The model under review builds one solid part; all positions refer to its coordinate system, in mm. A direction names the side the tool comes from. Coordinates: 2 decimals unless noted, no trailing zeros. Order: outer loops, then holes, each group sorted by start corner. A loop starts at its lowest first (then second) coordinate and runs counter-clockwise, first axis right, second up. Notation, with made-up numbers: M 42.25,45 L 97.25,45 A27 cw 97.25,84 Z; hole C -4,-23.75 d4. An arc over 180 degrees is marked long. Answer as CSV lines item,"result". Start each with the question number.
Q1. The part is to be moulded in two halves that separate along Y. For faces 4 (the face through (-39.8, -70.7, 37)), 5 (the face through (-25, 66, 28)), 6 (the face through (49.952, 56.985, 34.93)), say which applies: +Y half, -Y half, draft (parallel to the pull), parting line (faces both ways), or undercut.
Q2. Consider section A-A on z = 16.5. Write out the cut boundary in (x, y).
Q3. For P1, Ø3, axis at x = 14, z = -14.5, coming from the +Y side; P2, Ø10, axis at x = -6, z = 40, coming from the +Y side; P3, Ø11, axis at x = -9.5, z = 34, coming from the +Y side; P4, Ø3, axis at x = -52.5, y = 33.35, coming from the +Z side, all flat-tipped, find the tip position at first contact; note any pin that passes through.
Q4. Wall thickness on L1, parallel to Y at x = 0, z = -12; L2, parallel to Z at x = 36.5, y = 37; L3, parallel to Y at x = 52, z = 39: over which ranges is each line inside the solid? List them lowest first. Write a range as [from, to].
Q5. Consider section D-D on z = -10. Write out the cut boundary in (x, y).
Q6. Consider section C-C on x = 0. Write out the cut boundary in (y, z), and give its area (3 significant figures).
Q7. Machinability: for faces 1 (the face through (-3, -71.5, 23)), 2 (the face through (23.846, 7.509, -13.095)), 3 (the face through (0, 66, 25)), which of the approach directions +Z, -Z, +X, -X, +Y, -Y give a long, thin tool a straight path to every point of the face, cutting with its end or side? Answer none if there is none.
Q8. Consider section B-B on x = -52.5. Write out the cut boundary in (y, z).
from build123d import *

# Parameters (mm, degrees)
ESTRUSIONE_ESTRUSIONE1_DEPTH       = 30
ESTRUSIONE_ESTRUSIONE1_DEPTH_BACK  = 55
SCHIZZO1_R                         = 25
SCHIZZO1_R_2                       = 20
ESTRUSIONE_ESTRUSIONE2_DEPTH       = 10
ESTRUSIONE_ESTRUSIONE3_DEPTH       = 10
ESTRUSIONE_ESTRUSIONE5_DEPTH       = 42.5
TAGLIO_ESTRUSIONE1_DEPTH           = 26.5
SCHIZZO3D5_R                       = 2.5
TAGLIO_ESTRUSIONE2_DEPTH           = 35.5
SCHIZZO3D6_R                       = 4
TAGLIO_ESTRUSIONE3_DEPTH           = 3
ESTRUSIONE_ESTRUSIONE10_DEPTH      = 5
TAGLIO_ESTRUSIONE4_START           = -14
TAGLIO_ESTRUSIONE4_DEPTH           = 14
TAGLIO_ESTRUSIONE7_DEPTH           = 3
ESTRUSIONE_ESTRUSIONE11_START      = 30
ESTRUSIONE_ESTRUSIONE11_OUTLINE_R  = 4
ESTRUSIONE_ESTRUSIONE11_DEPTH      = 10
ESTRUSIONE_ESTRUSIONE12_DEPTH      = 10
ESTRUSIONE_ESTRUSIONE13_DEPTH      = 10
ESTRUSIONE_ESTRUSIONE14_DEPTH      = 10
TAGLIO_ESTRUSIONE11_DEPTH          = 80
SCHIZZO3D17_R                      = 4
TAGLIO_ESTRUSIONE12_DEPTH          = 3
TAGLIO_ESTRUSIONE13_START          = 30
TAGLIO_ESTRUSIONE13_OUTLINE_R      = 2.5
TAGLIO_ESTRUSIONE13_DEPTH          = 7
ESTRUSIONE_ESTRUSIONE15_DEPTH      = 5
ESTRUSIONE_ESTRUSIONE17_DEPTH      = 37.5
ESTRUSIONE_ESTRUSIONE17_DEPTH_BACK = 37.5


# Read off the part's stored shape, not the designer's step: Estrusione-Estrusione11, Taglio-Estrusione13
with BuildPart() as part:
    # Schizzo1 → Estrusione-Estrusione1 (new, two sides: drawn at the far end of the back side and taken through both)
    with BuildSketch(Plane.XY.offset(-ESTRUSIONE_ESTRUSIONE1_DEPTH_BACK)):
        Circle(SCHIZZO1_R)
        Circle(SCHIZZO1_R_2, mode=Mode.SUBTRACT)
    extrude(amount=ESTRUSIONE_ESTRUSIONE1_DEPTH + ESTRUSIONE_ESTRUSIONE1_DEPTH_BACK)

    # Schizzo3D1 → Estrusione-Estrusione2 (add)
    with BuildSketch(Plane(origin=(-37.75, 73.5, 30), x_dir=(0.4568693936855125, -0.889533786381064, 0), z_dir=(0, 0, -1))):
        Polygon((0, 0), (34.493639223, -67.159800872), (75.600538561, -73.870637396), (146.763241471, -37.321085901), (165.255105821, 0), (130.761466598, 67.159800872), (89.654567261, 73.870637396), (18.49186435, 37.321085901), align=None)
    extrude(amount=-ESTRUSIONE_ESTRUSIONE2_DEPTH)

    # Schizzo3D2 → Estrusione-Estrusione3 (add)
    with BuildSketch(Plane(origin=(62.5, 0, 30), x_dir=(-0.9968152785361251, -0.07974522228289001, 0), z_dir=(0, 0, 1))):
        Polygon((0, 0), (0.797452223, 9.968152785), (5.781528616, 9.569426674), (4.984076393, -0.398726111), align=None)
        Polygon((125.39936204, 0), (120.415285647, 0.398726111), (119.617833424, -9.569426674), (124.601909817, -9.968152785), align=None)
    extrude(amount=-ESTRUSIONE_ESTRUSIONE3_DEPTH)

    # Schizzo3D3 → Estrusione-Estrusione5 (add)
    with BuildSketch(Plane(origin=(35.227450684, -68.5, 30), x_dir=(-0.9974912873801348, -0.0707893466612134, 0), z_dir=(0, 0, 1))):
        Polygon((0, 0), (70.278150268, -4.987456437), (70.632097001, 0), (0.353946733, 4.987456437), align=None)
    extrude(amount=-ESTRUSIONE_ESTRUSIONE5_DEPTH)

    # Schizzo3D4 → Taglio-Estrusione1 (cut)
    with BuildSketch(Plane(origin=(32.75, -68.5, -12.5), x_dir=(-1, 0, 0), z_dir=(0, 1, 0))):
        with BuildLine():
            Line((0, 0), (65.5, 0))
            ThreePointArc((65.5, 0), (32.75, 32.75), (0, 0))
        make_face()
    extrude(amount=-TAGLIO_ESTRUSIONE1_DEPTH, mode=Mode.SUBTRACT)

    # Schizzo3D5 → Taglio-Estrusione2 (cut)
    with BuildSketch(Plane(origin=(-52.5, 33.353317087, 40), x_dir=(0.8440673996564301, -0.5362370975951146, 0), z_dir=(0, 0, -1))):
        with Locations(Location((0, 0, 0), (0, 0, 147.572152721))):
            Circle(SCHIZZO3D5_R)
        with Locations(Location((88.627076964, -56.304895247, 0), (0, 0, 147.572152721))):
            Circle(SCHIZZO3D5_R)
        with Locations(Location((124.397648864, 0, 0), (0, 0, 147.572152721))):
            Circle(SCHIZZO3D5_R)
        with Locations(Location((35.7705719, 56.304895247, 0), (0, 0, 147.572152721))):
            Circle(SCHIZZO3D5_R)
    extrude(amount=TAGLIO_ESTRUSIONE2_DEPTH, mode=Mode.SUBTRACT)

    # Schizzo3D6 → Taglio-Estrusione3 (cut)
    with BuildSketch(Plane(origin=(0, 73.5, 40), x_dir=(0, -1, 0), z_dir=(0, 0, -1))):
        with Locations(Location((40.146682913, 52.5, 0), (0, 0, 270))):
            Circle(SCHIZZO3D6_R)
        with Locations(Location((40.146682913, -52.5, 0), (0, 0, 270))):
            Circle(SCHIZZO3D6_R)
        with Locations(Location((106.853317087, -52.5, 0), (0, 0, 270))):
            Circle(SCHIZZO3D6_R)
        with Locations(Location((106.853317087, 52.5, 0), (0, 0, 270))):
            Circle(SCHIZZO3D6_R)
    extrude(amount=TAGLIO_ESTRUSIONE3_DEPTH, mode=Mode.SUBTRACT)

    # Schizzo3D7 → Estrusione-Estrusione10 (add)
    with BuildSketch(Plane(origin=(35.227450684, -73.5, -12.5), x_dir=(-0.8117651174974726, 0, 0.5839840700004706), z_dir=(0, 1, 0))):
        with BuildLine():
            Line((0, 0), (2.011108045, -1.446791734))
            ThreePointArc((2.011108045, -1.446791734), (47.721893936, 6.013037572), (55.181723242, -39.697748319))
            Line((55.181723242, -39.697748319), (57.192831287, -41.144540052))
            Line((57.192831287, -41.144540052), (82.012154262, -6.644522559))
            Line((82.012154262, -6.644522559), (84.059871804, -8.117651175))
            Line((84.059871804, -8.117651175), (89.899712504, 0))
            Line((89.899712504, 0), (28.611446133, 44.090797285))
            Line((28.611446133, 44.090797285), (22.771605433, 35.97314611))
            Line((22.771605433, 35.97314611), (24.819322975, 34.500017494))
            Line((24.819322975, 34.500017494), (0, 0))
        make_face()
    extrude(amount=-ESTRUSIONE_ESTRUSIONE10_DEPTH)

    # Schizzo3D8 → Taglio-Estrusione4 (cut)
    with BuildSketch(Plane(origin=(0, -78.5, 20.25), x_dir=(-0.707106781186551, 0, -0.7071067811865441), z_dir=(0, -1, 0)).offset(TAGLIO_ESTRUSIONE4_START)):
        with BuildLine():
            ThreePointArc((0, 46.315494168), (-0.707106781, -0.707106781), (46.315494168, 0))
            ThreePointArc((46.315494168, 0), (0, 0), (0, 46.315494168))
        make_face()
    extrude(amount=TAGLIO_ESTRUSIONE4_DEPTH, mode=Mode.SUBTRACT)

    # Schizzo3D9 → Taglio-Estrusione7 (cut)
    with BuildSketch(Plane(origin=(35.227450684, -68.5, -12.5), x_dir=(-0.8562730712113632, 0, 0.5165234046180869), z_dir=(0, -1, 0))):
        with BuildLine():
            Line((0, 0), (2.121374306, 1.279661262))
            ThreePointArc((2.121374306, 1.279661262), (13.749394894, 45.407843828), (58.20726047, 35.111944264))
            Line((58.20726047, 35.111944264), (60.328634776, 36.391605526))
            Line((60.328634776, 36.391605526), (82.280879472, 0))
            Line((82.280879472, 0), (21.952244696, -36.391605526))
            Line((21.952244696, -36.391605526), (0, 0))
        make_face()
    extrude(amount=TAGLIO_ESTRUSIONE7_DEPTH, mode=Mode.SUBTRACT)

    # Estrusione-Estrusione11 outline → Estrusione-Estrusione11 (add)
    with BuildSketch(Plane.XY.offset(ESTRUSIONE_ESTRUSIONE11_START)):
        with Locations((52.5, -33.353317087)):
            Circle(ESTRUSIONE_ESTRUSIONE11_OUTLINE_R)
        with Locations((-52.5, -33.353317087)):
            Circle(ESTRUSIONE_ESTRUSIONE11_OUTLINE_R)
    extrude(amount=ESTRUSIONE_ESTRUSIONE11_DEPTH)

    # Schizzo3D11 → Estrusione-Estrusione12 (add)
    with BuildSketch(Plane(origin=(-62.5, -40, 40), x_dir=(0.9979582700578467, -0.06386932928370219, 0), z_dir=(0, 0, -1))):
        Polygon((0, 0), (0.510954634, 7.98366616), (27.158436361, 36.840627497), (26.839089715, 31.850836147), align=None)
        Polygon((102.504285751, 32.018493137), (102.184939104, 27.028701786), (124.744783757, -7.98366616), (125.255738392, 0), align=None)
    extrude(amount=ESTRUSIONE_ESTRUSIONE12_DEPTH)

    # Schizzo3D12 → Estrusione-Estrusione13 (add)
    with BuildSketch(Plane(origin=(-37.75, -78.5, 40), x_dir=(0.9932296706390209, 0.11616721294023631, 0), z_dir=(0, 0, 1))):
        Polygon((0, 0), (-9.932296706, 1.161672129), (-8.770624577, 11.093968836), (1.161672129, 9.932296706), align=None)
        Polygon((74.988840133, -8.770624577), (84.92113684, -9.932296706), (86.082808969, 0), (76.150512263, 1.161672129), align=None)
    extrude(amount=-ESTRUSIONE_ESTRUSIONE13_DEPTH)

    # Schizzo3D15 → Estrusione-Estrusione14 (add)
    with BuildSketch(Plane(origin=(-49.75, -63.712121212, 40), x_dir=(0.9860632358712049, -0.16637095558783233, 0), z_dir=(0, 0, 1))):
        Polygon((0, 0), (4.627662115, -4.074759177), (2.768690441, -4.388409339), (4.432399997, -14.249041698), (98.601439022, 1.639384561), (96.937729467, 11.500016919), (95.078757792, 11.186366757), (98.113291969, 16.553910081), (100.573565494, 1.972126472), (100.906307405, 0), (2.793015436, -16.553910081), (2.460273525, -14.581783609), align=None)
    extrude(amount=-ESTRUSIONE_ESTRUSIONE14_DEPTH)

    # Schizzo3D16 → Taglio-Estrusione11 (cut)
    with BuildSketch(Plane(origin=(-49.75, -80.5, 40), x_dir=(0.9860632358712049, 0.16637095558783233, 0), z_dir=(0, 0, 1))):
        Polygon((0, 0), (1.972126472, -0.332741911), (4.35509632, 13.790870902), (2.793015436, 16.553910081), align=None)
        Polygon((98.113291969, -16.553910081), (96.141165497, -16.22116817), (98.524135346, -2.097555357), (100.906307405, 0), align=None)
    extrude(amount=-TAGLIO_ESTRUSIONE11_DEPTH, mode=Mode.SUBTRACT)

    # Schizzo3D17 → Taglio-Estrusione12 (cut)
    with BuildSketch(Plane(origin=(0, -80.5, 40), x_dir=(-0.9847878761773714, 0.17376086709631217, 0), z_dir=(0, 0, -1))):
        with Locations(Location((41.215356952, 0, 0), (0, 0, 169.993443701))):
            Circle(SCHIZZO3D17_R)
        with Locations(Location((-38.726539684, 14.10534554, 0), (0, 0, 169.993443701))):
            Circle(SCHIZZO3D17_R)
    extrude(amount=TAGLIO_ESTRUSIONE12_DEPTH, mode=Mode.SUBTRACT)

    # Taglio-Estrusione13 outline → Taglio-Estrusione13 (cut)
    with BuildSketch(Plane.XY.offset(TAGLIO_ESTRUSIONE13_START)):
        with Locations((-40.588383838, -73.338383838)):
            Circle(TAGLIO_ESTRUSIONE13_OUTLINE_R)
        with Locations((40.588383838, -73.338383838)):
            Circle(TAGLIO_ESTRUSIONE13_OUTLINE_R)
    extrude(amount=TAGLIO_ESTRUSIONE13_DEPTH, mode=Mode.SUBTRACT)

    # Schizzo3D19 → Estrusione-Estrusione15 (add)
    with BuildSketch(Plane(origin=(0, 68.5, 30), x_dir=(0.9805806756909201, -0.19611613513818418, 0), z_dir=(0, 0, -1))):
        Polygon((0, 0), (-24.514516892, 4.902903378), (-23.533936217, 9.805806757), (25.495097568, 0), (24.514516892, -4.902903378), align=None)
    extrude(amount=ESTRUSIONE_ESTRUSIONE15_DEPTH)

    # Schizzo3D21 → Estrusione-Estrusione17 (add, two sides: drawn at the far end of the back side and taken through both)
    with BuildSketch(Plane(origin=(0, 73.5, 40), x_dir=(0, 0.4472135954999578, 0.8944271909999159), z_dir=(1, 0, 0)).offset(-ESTRUSIONE_ESTRUSIONE17_DEPTH_BACK)):
        Polygon((0, 0), (38.013155617, 0), (35.329874044, 5.366563146), (-2.683281573, 5.366563146), align=None)
    extrude(amount=ESTRUSIONE_ESTRUSIONE17_DEPTH + ESTRUSIONE_ESTRUSIONE17_DEPTH_BACK)


solid = part.part
Evaluation:
1,face 4,"undercut"
1,face 5,"draft"
1,face 6,"+Y half"
2,outline,"M -35.23,-78.5 L -16.99,-78.5 L -16.99,-71.5 L -35.23,-71.5 Z; C 0,0 d50; M 16.99,-78.5 L 35.23,-78.5 L 35.23,-71.5 L 16.99,-71.5 Z; hole C 0,0 d40"
3,P1,"stops at y = 21.65"
3,P2,"stops at y = 76"
3,P3,"stops at y = 73.5"
3,P4,"passes through"
4,L1,"y = [-25, -20], [20, 25]"
4,L2,"z = [30, 40]"
4,L3,"y = [-60.94, 29.38], [37.32, 54.21]"
5,outline,"M -35.23,-78.5 L -32.73,-78.5 L -32.73,-71.5 L -35.23,-71.5 Z; C 0,0 d50; M 32.73,-78.5 L 35.23,-78.5 L 35.23,-71.5 L 32.73,-71.5 Z; hole C 0,0 d40"
6,outline,"M -80.5,30 L -78.5,30 L -78.5,21.25 L -71.5,21.25 L -71.5,30 L -25,30 L -25,-55 L -20,-55 L -20,30 L 20,30 L 20,-55 L 25,-55 L 25,30 L 63.5,30 L 63.5,25 L 68.5,25 L 68.5,30 L 73.5,30 L 73.5,40 L 90.5,74 L 84.5,74 L 67.5,40 L -80.5,40 Z"
6,area,"2,680 mm²"
7,face 1,"-Z, +X, -X"
7,face 2,"-Z"
7,face 3,"-Z, +X, -X, +Y"
8,outline,"M -60.32,30 L 30.85,30 L 30.85,37 L 29.35,37 L 29.35,40 L -60.32,40 Z; M 35.85,30 L 53.54,30 L 53.54,40 L 37.35,40 L 37.35,37 L 35.85,37 Z"
